```python
from build123d import *

# Parameters (mm, degrees)
SKETCH1_W           = 90
SKETCH1_H           = 60
BOSS_EXTRUDE1_DEPTH = 40
SKETCH2_W           = 40.3
SKETCH2_H           = 38
CUT_EXTRUDE1_DEPTH  = 61
SKETCH3_R           = 4.1
CUT_EXTRUDE2_DEPTH  = 41
CHAMFER1_SIZE       = 1


with BuildPart() as part:
    # Sketch1 → Boss-Extrude1 (new body)
    with BuildSketch(Plane(origin=(0, 0, 0), x_dir=(1, 0, 0), z_dir=(0, 1, 0))):
        Rectangle(SKETCH1_W, SKETCH1_H)
    extrude(amount=BOSS_EXTRUDE1_DEPTH)

    # Sketch2 → Cut-Extrude1 (cut, through all)
    with BuildSketch(Plane.XY.offset(30)):
        with Locations((0, 40)):
            Rectangle(SKETCH2_W, SKETCH2_H)
    extrude(amount=-CUT_EXTRUDE1_DEPTH, mode=Mode.SUBTRACT)

    # Sketch3 → Cut-Extrude2 (cut, through all)
    with BuildSketch(Plane.XZ):
        with Locations((-35, 15)):
            Circle(SKETCH3_R)
        with Locations((-35, -15)):
            Circle(SKETCH3_R)
        with Locations((35, -14.217273236)):
            Circle(SKETCH3_R)
        with Locations((35, 15)):
            Circle(SKETCH3_R)
    extrude(amount=-CUT_EXTRUDE2_DEPTH, mode=Mode.SUBTRACT)

    # Chamfer1
    chamfer1_edges = [part.edges().sort_by_distance(p)[0] for p in [
        (20.15, 40, 0),
        (-20.15, 40, 0),
    ]]
    chamfer(chamfer1_edges, length=CHAMFER1_SIZE)


solid = part.part
```
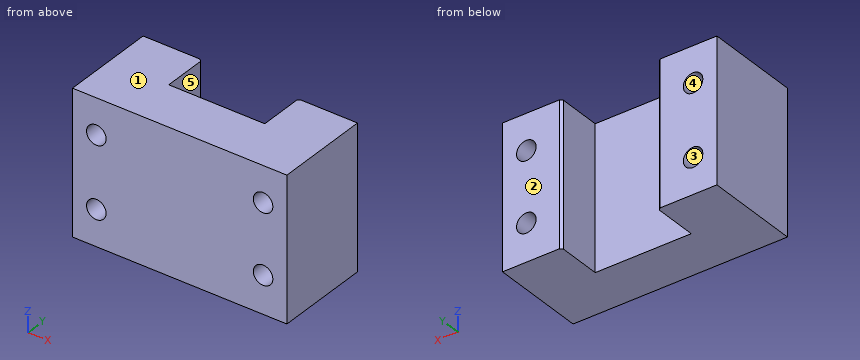
Design review of the part built by this model. Coordinates are the model's own, in mm. Face numbers are marked on the shaded views. A direction names the side the tool comes from. Coordinates: 2 decimals unless noted, no trailing zeros. Order: outer loops, then holes, each group sorted by start corner. A loop starts at its lowest first (then second) coordinate and runs counter-clockwise, first axis right, second up. Notation, with made-up numbers: M 16,14 L 74,14 A18 ccw 74,25 Z; hole C -23.75,35 d8. An arc over 180 degrees is marked long. Answer as a JSON object with one key per item and string values. Group by question number.
1) Add section B-B, the plane x = -35. Write out the cut boundary in (y, z), then the cut area to 3 significant figures.
2) For pin 1 (9.5 mm diameter, centred on x = -35, z = 15, fed in from +Y), flat-tipped, find the tip position at first contact; note if it passes through.
3) Tool access review of the marked faces 4 and 5: name each direction out of +Z, -Z, +X, -X, +Y, -Y from which nothing blocks a thin tool from reaching the whole face with its end or side.
4) Add section D-D, the plane y = 10. Write out the cut boundary in (x, z), then the cut area to 3 significant figures.
5) Mouldability with a two-part tool opening along Z and no side actions: class the marked faces 1, 2 and 3 as pulls with the +Z half, pulls with the -Z half, needs draft (parallel to the pull), parting line crosses it, or undercut.
6) Wall thickness on L1, parallel to Z at x = -35, y = 24.5; L2, parallel to Z at x = 35, y = 32; L3, parallel to X at y = 37, z = 3: over which ranges is each line inside the solid? List them lowest first.
7) Add section C-C, the plane y = 26. Write out the cut boundary in (x, z), then the cut area to 3 significant figures.
8) Add section A-A, the plane z = 15. Write out the cut boundary in (x, y).
Computed values:
{
 "1": {"outline": "M 0,-30 L 40,-30 L 40,-19.1 L 0,-19.1 Z; M 0,-10.9 L 40,-10.9 L 40,10.9 L 0,10.9 Z; M 0,19.1 L 40,19.1 L 40,30 L 0,30 Z", "area": "1,740 mm^2"},
 "2": {"pin 1": "stops at y = 40"},
 "3": {"face 4": "+Y, -Y", "face 5": "+Z, -Z, +Y"},
 "4": {"outline": "M -45,-30 L 45,-30 L 45,30 L -45,30 Z; hole C -35,-15 d8.2; hole C -35,15 d8.2; hole C 35,-14.22 d8.2; hole C 35,15 d8.2", "area": "5,190 mm^2"},
 "5": {"face 1": "pulls with the +Z half", "face 2": "needs draft", "face 3": "undercut"},
 "6": {"L1": "z = -30 to -19.1, -10.9 to 10.9, 19.1 to 30", "L2": "z = -30 to -18.32, -10.12 to 10.9, 19.1 to 30", "L3": "x = -45 to -20.15, 20.15 to 45"},
 "7": {"outline": "M -45,-30 L -20.15,-30 L -20.15,30 L -45,30 Z; M 20.15,-30 L 45,-30 L 45,30 L 20.15,30 Z; hole C -35,-15 d8.2; hole C -35,15 d8.2; hole C 35,-14.22 d8.2; hole C 35,15 d8.2", "area": "2,770 mm^2"},
 "8": {"outline": "M -45,0 L -39.1,0 L -39.1,40 L -45,40 Z; M -30.9,0 L 30.9,0 L 30.9,40 L 21.15,40 L 20.15,39 L 20.15,21 L -20.15,21 L -20.15,39 L -21.15,40 L -30.9,40 Z; M 39.1,0 L 45,0 L 45,40 L 39.1,40 Z"}
}
